Input: part model. Units: mm. Frame: model coordinates. Face numbers are marked on the shaded views. A direction names the side the tool comes from. Round coordinates to 2 decimals unless told otherwise and drop trailing zeros. Order: outer loops, then holes, each group sorted by start corner. A loop starts at its lowest first (then second) coordinate and runs counter-clockwise, first axis right, second up. Notation, with made-up numbers: (-15.5, -34.5) -> (-11.5, -34.5) arc R22 cw to (-11.5, -22.5) -> close; hole circle Ø3 at (26.5, 85.5). An arc over 180 degrees is marked (long way). Use a Markdown table: item, result.
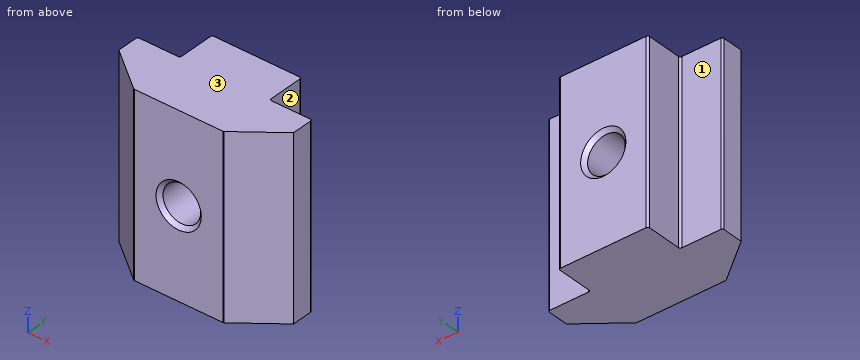
from build123d import *

# Parameters (mm, degrees)
EXTRUDE_1_DEPTH = 10
FILLET_1_R      = 0.2


with BuildPart() as part:
    # Эскиз1 → Бобышка-Вытянуть1 (new body, symmetric)
    with BuildSketch(Plane.XY):
        Polygon((5, 0), (-5, 0), (-5, -4.3), (-9.75, -4.3), (-9.75, -6.8), (-5, -10.5), (5, -10.5), (9.75, -6.8), (9.75, -4.3), (5, -4.3), align=None)
    extrude(amount=EXTRUDE_1_DEPTH, both=True)

    # Эскиз4 → Отверстие обработанное метчиком M54 (revolve, cut)
    with BuildSketch(Plane(origin=(0, 0, 0), x_dir=(0, 0, 1), z_dir=(1, 0, 0))):
        Polygon((0, 0), (0, 10.5), (2.525, 10.5), (2.1, 10.075), (2.1, 0.425), (2.525, 0), align=None)
    revolve(axis=Axis((0, 6.35, 0), (0, -1, 0)), mode=Mode.SUBTRACT)

    # Скругление1
    fillet_1_edges = [part.edges().sort_by_distance(p)[0] for p in [
        (-5, 0, 0),
        (5, 0, 0),
        (5, -4.3, 0),
        (9.75, -4.3, 0),
        (5, -10.5, 0),
        (-5, -10.5, 0),
        (-9.75, -4.3, 0),
        (-5, -4.3, 0),
    ]]
    fillet(fillet_1_edges, radius=FILLET_1_R)


solid = part.part
1) Cut plane D-D on z = -5.25. Return loops of the section in (x, y), and give its area (3 significant figures).
Answer key:
| item | result |
|---|---|
| outline | (-9.75, -6.8) -> (-5.05, -10.46) arc R0.2 ccw to (-4.93, -10.5) -> (4.93, -10.5) arc R0.2 ccw to (5.05, -10.46) -> (9.75, -6.8) -> (9.75, -4.5) arc R0.2 ccw to (9.55, -4.3) -> (5.2, -4.3) arc R0.2 cw to (5, -4.1) -> (5, -0.2) arc R0.2 ccw to (4.8, 0) -> (-4.8, 0) arc R0.2 ccw to (-5, -0.2) -> (-5, -4.1) arc R0.2 cw to (-5.2, -4.3) -> (-9.55, -4.3) arc R0.2 ccw to (-9.75, -4.5) -> close |
| area | 146 mm^2 |
2) Ray query, probe 1 along X at (y, z) = (-3.25, 0); probe 2 along X at (y, z) = (-5, 0); probe 3 along Z at (x, y) = (0, -3.5). Return the intervals inside material, ascending.
Answer key:
| item | result |
|---|---|
| probe 1 | x = -5 to -2.1, 2.1 to 5 |
| probe 2 | x = -9.75 to -2.1, 2.1 to 9.75 |
| probe 3 | z = -10 to -2.1, 2.1 to 10 |
3) Contact query for flat-ended pins moving along their axis: P1, Ø5, axis at x = -7, z = -5, coming from the +Y side; P2, Ø2, axis at x = 6.5, z = 0.5, coming from the +Y side; P3, Ø3, axis at y = -2.5, z = -3, coming from the -X side. Output: stop coordinate, or through.
Answer key:
| item | result |
|---|---|
| P1 | stops at y = 0 |
| P2 | stops at y = -4.3 |
| P3 | stops at x = -5 |
4) Set-up query: the marked faces 1, 2 and 3. Return all of +Z, -Z, +X, -X, +Y, -Y with unobstructed straight access to the full face (end or side cutting, diameter ignored); none if empty.
Answer key:
| item | result |
|---|---|
| face 1 | +Z, -Z, -X, +Y |
| face 2 | +Z, -Z, +X, +Y |
| face 3 | +Z, +X, -X, +Y, -Y |
5) Cut plane C-C on y = -6.5. Return loops of the section in (x, z), and give its area (3 significant figures).
Answer key:
| item | result |
|---|---|
| outline | (-9.75, -10) -> (9.75, -10) -> (9.75, 10) -> (-9.75, 10) -> close; hole circle Ø4.2 at (0, 0) |
| area | 376 mm^2 |
6) Cut plane B-B on z = 0. Return loops of the section in (x, y) (3 decimals), and give its area (3 significant figures).
Answer key:
| item | result |
|---|---|
| outline | (-9.75, -6.8) -> (-5.054, -10.458) arc R0.2 ccw to (-4.931, -10.5) -> (-2.525, -10.5) -> (-2.1, -10.075) -> (-2.1, -0.425) -> (-2.525, 0) -> (-4.8, 0) arc R0.2 ccw to (-5, -0.2) -> (-5, -4.1) arc R0.2 cw to (-5.2, -4.3) -> (-9.55, -4.3) arc R0.2 ccw to (-9.75, -4.5) -> close; (2.1, -10.075) -> (2.525, -10.5) -> (4.931, -10.5) arc R0.2 ccw to (5.054, -10.458) -> (9.75, -6.8) -> (9.75, -4.5) arc R0.2 ccw to (9.55, -4.3) -> (5.2, -4.3) arc R0.2 cw to (5, -4.1) -> (5, -0.2) arc R0.2 ccw to (4.8, 0) -> (2.525, 0) -> (2.1, -0.425) -> close |
| area | 102 mm^2 |
7) Cut plane A-A on x = 0. Return loops of the section in (y, z) (3 decimals), and give its area (3 significant figures).
Answer key:
| item | result |
|---|---|
| outline | (-10.5, -10) -> (0, -10) -> (0, -2.525) -> (-0.425, -2.1) -> (-10.075, -2.1) -> (-10.5, -2.525) -> close; (-10.5, 2.525) -> (-10.075, 2.1) -> (-0.425, 2.1) -> (0, 2.525) -> (0, 10) -> (-10.5, 10) -> close |
| area | 166 mm^2 |
